Could you check a few things on this model? Use its own coordinates, in mm. Face numbers are marked on the shaded views. Coordinates: 2 decimals unless noted, no trailing zeros. Loops run counter-clockwise (first coordinate to the right, second up) from the corner with the lowest first, then second, coordinate; pieces in that order, holes last. Notation, with made-up numbers: (-23, 11.25) -> (-7, 11.25) arc R16 ccw to (-7, 19.25) -> close; hole circle Ø5 at (23, 82.25). An arc over 180 degrees is marked (long way). One line per question, with ' | ' between items.
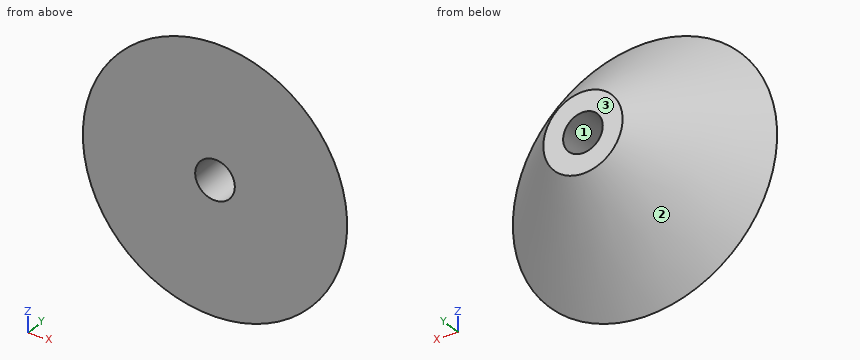
from build123d import *

# Parameters (mm, degrees)
SKETCH1_R           = 10
BOSS_EXTRUDE1_DEPTH = 7
CHAMFER1_SIZE       = 7
SKETCH2_R           = 1.5
CUT_EXTRUDE1_DEPTH  = 16.779733838


with BuildPart() as part:
    # Sketch1 → Boss-Extrude1 (new body)
    with BuildSketch(Plane(origin=(0, 0, 0), x_dir=(1, 0, 0), z_dir=(0, 1, 0))):
        with Locations(Location((0, 0, 0), (0, 0, 270))):
            Circle(SKETCH1_R)
    extrude(amount=BOSS_EXTRUDE1_DEPTH)

    # Chamfer1
    chamfer1_edges = [part.edges().sort_by_distance(p)[0] for p in [
        (0, 7, -10),
    ]]
    chamfer(chamfer1_edges, length=CHAMFER1_SIZE - 0.0001)  # a hair under: the kernel refuses the full size

    # Sketch2 → Cut-Extrude1 (cut, through all)
    with BuildSketch(Plane(origin=(0, 7, 0), x_dir=(1, 0, 0), z_dir=(0, 1, 0))):
        with Locations(Location((0, 0, 0), (0, 0, 270))):
            Circle(SKETCH2_R)
    extrude(amount=-CUT_EXTRUDE1_DEPTH, mode=Mode.SUBTRACT)


solid = part.part
1) I need wall thicknesses on line 1 along X through (y, z) = (1.75, 0); line 2 along X through (y, z) = (4, 0); line 3 along Y through (x, z) = (-6.75, 3.75). Which ranges of each line are inside material? Lowest first, please. Write a range as from..to.
Data:
line 1: -8.25..-1.5, 1.5..8.25 | line 2: -6..-1.5, 1.5..6 | line 3: 0..2.28
2) If we section it at C-C on y = 4: Please give me the cut outline in (x, z), and give its area (3 significant figures).
Data:
outline: circle Ø12 at (0, 0); hole circle Ø3 at (0, 0) | area: 106 mm²
3) We'd pull the mould along Z, two halves only. Please class the marked faces 1, 2 and 3: pulls with the +Z half, pulls with the -Z half, needs draft (parallel to the pull), parting line crosses it, or undercut.
Data:
face 1: undercut | face 2: parting line crosses it | face 3: needs draft
4) I'm going to push flat-ended pins straight in: pin 1 Ø2 at (y, z) = (5.5, 1.5) entering from +X; pin 2 Ø2.5 at (x, z) = (0, 0) entering from +Y; pin 3 Ø1 at (y, z) = (3, -1.5) entering from +X; pin 4 Ø2 at (y, z) = (4.5, 5) entering from -X. Where does each tip first touch, or does it pass through?
Data:
pin 1: x = 5.32 | pin 2: through | pin 3: x = 7.36 | pin 4: x = -4.51
